For this review, take the finished solid that the model builds, in its own axes (mm). Face numbers are marked on the shaded views. A direction names the side the tool comes from. Round coordinates to 2 decimals unless told otherwise and drop trailing zeros. Order: outer loops, then holes, each group sorted by start corner. A loop starts at its lowest first (then second) coordinate and runs counter-clockwise, first axis right, second up. Notation, with made-up numbers: (68, 78) -> (75, 78) arc R10 cw to (75, 84) -> close; hole circle Ø10 at (32.5, 38). An arc over 180 degrees is marked (long way). Use a Markdown table: item, result. Add a question column.
1) Consider section B-B (z = 7.75). Give the number of separate pieces and of enclosed holes in the cut face, plus the area to 3 significant figures.
2) Consider section C-C (x = -15). State the section outline as (y, z) points.
3) Consider section D-D (z = 1.5). State the section outline as (x, y) points.
4) Clearance check with a flat-ended pin moving along its axis: P1, Ø7.5, axis at x = -25.12, y = -12.5, coming from the -Z side. State where the tip first meets the part, or that it passes through.
5) Machinability: for the marked faces 1, 2 and 3, which of the approach directions +Z, -Z, +X, -X, +Y, -Y give a long, thin tool a straight path to every point of the face, cutting with its end or side? Answer none if there is none.
6) Consider section A-A (y = 37.5). State the section outline as (x, z) points.
7) Wall thickness on line 1 along Y through (x, z) = (-12.5, 3.65); line 2 along Y through (x, z) = (-39, 1.25); line 3 along X through (y, z) = (-7, 6): over which ranges is each line inside the solid? List them lowest first. Write a range as [from, to].
8) Draft analysis for pull direction Y (two halves, no side actions). For the marked faces 4, 5 and 6, state which applies: pulls with the +Y half, pulls with the -Y half, needs draft (parallel to the pull), parting line crosses it, or undercut.
Autodesk Inventor part; units mm, degrees
ref_plane "YZ Plane" through (0, 0, 0) normal (1, 0, 0) x (0, 1, 0)
ref_plane "XZ Plane" through (0, 0, 0) normal (0, 1, 0) x (-1, 0, 0)
ref_plane "XY Plane" through (0, 0, 0) normal (0, 0, 1) x (1, 0, 0)
sketch "Sketch1" plane through (0, 0, 0) normal (0, 0, 1) x (1, 0, 0)
  line L0 (-6.25, 43.75) -> (-43.75, 43.75)
  line L1 (-43.75, 43.75) -> (-43.75, -18.75)
  line L2 (-43.75, -18.75) -> (-6.25, -18.75)
  line L3 (-6.25, -18.75) -> (-6.25, 43.75)
  circle A0 centre (-12.5, 37.5) radius 3.25
  circle A1 centre (-37.5, 37.5) radius 3.25
  circle A2 centre (-37.5, -12.5) radius 3.25
  line L4 (-12.5, 37.5) -> (-6.25, 37.5)
  line L5 (-12.5, -12.5) -> (-12.5, -18.75)
  line L6 (-37.5, 37.5) -> (-37.5, 43.75)
  line L7 (-37.5, -12.5) -> (-43.75, -12.5)
  circle A3 centre (-12.5, -12.5) radius 3.25
  circle A4 centre (-25.1179, 37.5) radius 3.25
  circle A5 centre (-25.1179, -12.5) radius 3.25
  line L8 (-25.1179, 31.7265) -> (-30.1179, 34.6132)
  line L9 (-30.1179, 34.6132) -> (-30.1179, 40.3868)
  line L10 (-30.1179, 40.3868) -> (-25.1179, 43.2735)
  line L11 (-25.1179, 43.2735) -> (-20.1179, 40.3868)
  line L12 (-20.1179, 40.3868) -> (-20.1179, 34.6132)
  line L13 (-20.1179, 34.6132) -> (-25.1179, 31.7265)
  line L14 (-25.1179, -6.7265) -> (-20.1179, -9.6132)
  line L15 (-20.1179, -9.6132) -> (-20.1179, -15.3868)
  line L16 (-20.1179, -15.3868) -> (-25.1179, -18.2735)
  line L17 (-25.1179, -18.2735) -> (-30.1179, -15.3868)
  line L18 (-30.1179, -15.3868) -> (-30.1179, -9.6132)
  line L19 (-30.1179, -9.6132) -> (-25.1179, -6.7265)
  point P0 (0, 0)
  point P1 (-20.1179, 37.5)
  point P2 (-30.1179, 37.5)
  point P3 (-20.1179, -12.5)
  point P4 (-30.1179, -12.5)
  dimension "d1" = 6.25
  dimension "d42" = 6.5
  dimension "d43" = 6.5
  dimension "d44" = 10
  dimension "d45" = 10
extrude "Extrusion1" add sketch "Sketch1" along normal blind 10 contours L3 L2 L1 L0 | L8 L9 L10 L11 L12 L13 | L14 L15 L16 L17 L18 L19
sketch "Sketch2" plane through (0, 0, 10) normal (0, 0, 1) x (1, 0, 0)
  circle A0 centre (-12.5, 37.5) radius 3.25
  circle A1 centre (-37.5, 37.5) radius 3.25
  circle A2 centre (-37.5, -12.5) radius 3.25
  circle A3 centre (-12.5, -12.5) radius 3.25
  line L0 (-12.5, 31.7265) -> (-17.5, 34.6132)
  line L1 (-17.5, 34.6132) -> (-17.5, 40.3868)
  line L2 (-17.5, 40.3868) -> (-12.5, 43.2735)
  line L3 (-12.5, 43.2735) -> (-7.5, 40.3868)
  line L4 (-7.5, 40.3868) -> (-7.5, 34.6132)
  line L5 (-7.5, 34.6132) -> (-12.5, 31.7265)
  line L6 (-37.5, 31.7265) -> (-42.5, 34.6132)
  line L7 (-42.5, 34.6132) -> (-42.5, 40.3868)
  line L8 (-42.5, 40.3868) -> (-37.5, 43.2735)
  line L9 (-37.5, 43.2735) -> (-32.5, 40.3868)
  line L10 (-32.5, 40.3868) -> (-32.5, 34.6132)
  line L11 (-32.5, 34.6132) -> (-37.5, 31.7265)
  line L12 (-32.5208, -15.4225) -> (-37.5413, -18.2734)
  line L13 (-37.5413, -18.2734) -> (-42.5205, -15.3509)
  line L14 (-42.5205, -15.3509) -> (-42.4792, -9.5775)
  line L15 (-42.4792, -9.5775) -> (-37.4587, -6.7266)
  line L16 (-37.4587, -6.7266) -> (-32.4795, -9.6491)
  line L17 (-32.4795, -9.6491) -> (-32.5208, -15.4225)
  line L18 (-12.5, -6.7265) -> (-7.5, -9.6132)
  line L19 (-7.5, -9.6132) -> (-7.5, -15.3868)
  line L20 (-7.5, -15.3868) -> (-12.5, -18.2735)
  line L21 (-12.5, -18.2735) -> (-17.5, -15.3868)
  line L22 (-17.5, -15.3868) -> (-17.5, -9.6132)
  line L23 (-17.5, -9.6132) -> (-12.5, -6.7265)
  dimension "d33" = 10
  dimension "d34" = 10
  dimension "d35" = 10
  dimension "d36" = 10
extrude "Extrusion2" cut sketch "Sketch2" against normal blind 5
extrude "Extrusion5" cut sketch "Sketch1" along normal blind 5 contours L8 L9 L10 L11 L12 L13 | L14 L15 L16 L17 L18 L19
properties part number "print_head_mount"
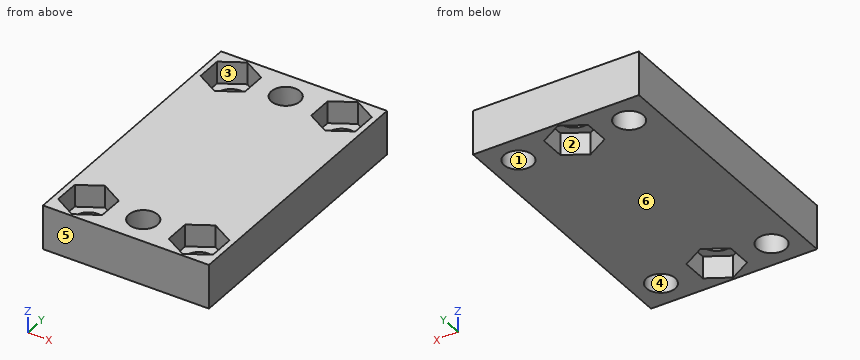
Results list:
| question | item | result |
|---|---|---|
| 1 | separate pieces | 1 |
| 1 | enclosed holes | 6 |
| 1 | area | 1,930 mm2 |
| 2 | outline | (-18.75, 0) -> (-14.58, 0) -> (-14.58, 5) -> (-16.83, 5) -> (-16.83, 10) -> (-18.75, 10) -> close; (-10.42, 0) -> (35.42, 0) -> (35.42, 5) -> (33.17, 5) -> (33.17, 10) -> (-8.17, 10) -> (-8.17, 5) -> (-10.42, 5) -> close; (39.58, 0) -> (43.75, 0) -> (43.75, 10) -> (41.83, 10) -> (41.83, 5) -> (39.58, 5) -> close |
| 3 | outline | (-43.75, -18.75) -> (-6.25, -18.75) -> (-6.25, 43.75) -> (-43.75, 43.75) -> close; hole circle Ø6.5 at (-37.5, -12.5); hole circle Ø6.5 at (-37.5, 37.5); hole (-30.12, -15.39) -> (-25.12, -18.27) -> (-20.12, -15.39) -> (-20.12, -9.61) -> (-25.12, -6.73) -> (-30.12, -9.61) -> close; hole (-30.12, 34.61) -> (-25.12, 31.73) -> (-20.12, 34.61) -> (-20.12, 40.39) -> (-25.12, 43.27) -> (-30.12, 40.39) -> close; hole circle Ø6.5 at (-12.5, -12.5); hole circle Ø6.5 at (-12.5, 37.5) |
| 4 | P1 | z = 5 |
| 5 | face 1 | +Z, -Z |
| 5 | face 2 | -Z |
| 5 | face 3 | +Z |
| 6 | outline | (-43.75, 0) -> (-40.75, 0) -> (-40.75, 5) -> (-42.5, 5) -> (-42.5, 10) -> (-43.75, 10) -> close; (-34.25, 0) -> (-30.12, 0) -> (-30.12, 5) -> (-28.37, 5) -> (-28.37, 10) -> (-32.5, 10) -> (-32.5, 5) -> (-34.25, 5) -> close; (-21.87, 5) -> (-20.12, 5) -> (-20.12, 0) -> (-15.75, 0) -> (-15.75, 5) -> (-17.5, 5) -> (-17.5, 10) -> (-21.87, 10) -> close; (-9.25, 0) -> (-6.25, 0) -> (-6.25, 10) -> (-7.5, 10) -> (-7.5, 5) -> (-9.25, 5) -> close |
| 7 | line 1 | [-18.75, -15.75], [-9.25, 34.25], [40.75, 43.75] |
| 7 | line 2 | [-18.75, -15.38], [-9.62, 34.62], [40.38, 43.75] |
| 7 | line 3 | [-43.75, -37.94], [-36.99, -12.97], [-12.03, -6.25] |
| 8 | face 4 | undercut |
| 8 | face 5 | pulls with the -Y half |
| 8 | face 6 | needs draft |
